For this review, take the finished solid that the model builds, in its own axes (mm). A direction names the side the tool comes from. Give positions to 0.01 mm unless a question says otherwise; leave off trailing zeros. Write each loop counter-clockwise with the first axis right and the second up, starting at its lowest first coordinate (ties: lowest second). Pieces come first, ordered by that corner, then holes. Notation, with made-up numbers: (87, 16.5) -> (111, 16.5) arc R21 ccw to (111, 21.5) -> close; hole circle Ø11 at (25.5, 22). An arc over 180 degrees is marked (long way). Return JSON: item names as keys, results as strings.
from build123d import *

# Parameters (mm, degrees)
SKETCH1_R           = 2.5
BOSS_EXTRUDE1_DEPTH = 283


with BuildPart() as part:
    # Sketch1 → Boss-Extrude1 (new body)
    with BuildSketch(Plane.XY):
        with BuildLine():
            Line((14.316619525, 10.387216168), (13.029112559, 10.387216168))
            Line((13.029112559, 10.387216168), (13.029112559, 12.855371932))
            Line((13.029112559, 12.855371932), (11.656738465, 12.855371932))
            Line((11.656738465, 12.855371932), (11.656738465, 12.336659272))
            Line((11.656738465, 12.336659272), (11.229112559, 12.336659272))
            Line((11.229112559, 12.336659272), (11.229112559, 7.521203168))
            ThreePointArc((11.229112559, 7.521203168), (11.668452387, 6.460542996), (12.729112559, 6.021203168))
            Line((12.729112559, 6.021203168), (17.624436699, 6.021203168))
            Line((17.624436699, 6.021203168), (17.624436699, 6.382997838))
            Line((17.624436699, 6.382997838), (18.129112559, 6.382997838))
            Line((18.129112559, 6.382997838), (18.129112559, 7.755371932))
            Line((18.129112559, 7.755371932), (15.794230869, 7.755371932))
            Line((15.794230869, 7.755371932), (15.794230869, 9.042878898))
            Line((15.794230869, 9.042878898), (18.806723903, 12.055371932))
            Line((18.806723903, 12.055371932), (23.784775289, 12.055371932))
            Line((23.784775289, 12.055371932), (26.797268323, 9.042878898))
            Line((26.797268323, 9.042878898), (26.797268323, 7.755371932))
            Line((26.797268323, 7.755371932), (24.329112559, 7.755371932))
            Line((24.329112559, 7.755371932), (24.329112559, 6.382997838))
            Line((24.329112559, 6.382997838), (24.847825219, 6.382997838))
            Line((24.847825219, 6.382997838), (24.847825219, 6.021203168))
            Line((24.847825219, 6.021203168), (29.729112559, 6.021203168))
            ThreePointArc((29.729112559, 6.021203168), (30.789772731, 6.460542996), (31.229112559, 7.521203168))
            Line((31.229112559, 7.521203168), (31.229112559, 12.350696072))
            Line((31.229112559, 12.350696072), (30.801486653, 12.350696072))
            Line((30.801486653, 12.350696072), (30.801486653, 12.855371932))
            Line((30.801486653, 12.855371932), (29.429112559, 12.855371932))
            Line((29.429112559, 12.855371932), (29.429112559, 10.520490242))
            Line((29.429112559, 10.520490242), (28.141605593, 10.520490242))
            Line((28.141605593, 10.520490242), (25.129112559, 13.532983276))
            Line((25.129112559, 13.532983276), (25.129112559, 18.511034662))
            Line((25.129112559, 18.511034662), (28.141605593, 21.523527696))
            Line((28.141605593, 21.523527696), (29.429112559, 21.523527696))
            Line((29.429112559, 21.523527696), (29.429112559, 19.055371932))
            Line((29.429112559, 19.055371932), (30.801486653, 19.055371932))
            Line((30.801486653, 19.055371932), (30.801486653, 19.574084592))
            Line((30.801486653, 19.574084592), (31.229112559, 19.574084592))
            Line((31.229112559, 19.574084592), (31.229112559, 24.389540696))
            ThreePointArc((31.229112559, 24.389540696), (30.789772731, 25.450200868), (29.729112559, 25.889540696))
            Line((29.729112559, 25.889540696), (24.833788419, 25.889540696))
            Line((24.833788419, 25.889540696), (24.833788419, 25.527746026))
            Line((24.833788419, 25.527746026), (24.329112559, 25.527746026))
            Line((24.329112559, 25.527746026), (24.329112559, 24.155371932))
            Line((24.329112559, 24.155371932), (26.663994249, 24.155371932))
            Line((26.663994249, 24.155371932), (26.663994249, 22.867864966))
            Line((26.663994249, 22.867864966), (23.651501215, 19.855371932))
            Line((23.651501215, 19.855371932), (18.673449829, 19.855371932))
            Line((18.673449829, 19.855371932), (15.660956795, 22.867864966))
            Line((15.660956795, 22.867864966), (15.660956795, 24.155371932))
            Line((15.660956795, 24.155371932), (18.129112559, 24.155371932))
            Line((18.129112559, 24.155371932), (18.129112559, 25.527746026))
            Line((18.129112559, 25.527746026), (17.610399899, 25.527746026))
            Line((17.610399899, 25.527746026), (17.610399899, 25.889540696))
            Line((17.610399899, 25.889540696), (12.729112559, 25.889540696))
            ThreePointArc((12.729112559, 25.889540696), (11.668452387, 25.450200868), (11.229112559, 24.389540696))
            Line((11.229112559, 24.389540696), (11.229112559, 19.560047792))
            Line((11.229112559, 19.560047792), (11.656738465, 19.560047792))
            Line((11.656738465, 19.560047792), (11.656738465, 19.055371932))
            Line((11.656738465, 19.055371932), (13.029112559, 19.055371932))
            Line((13.029112559, 19.055371932), (13.029112559, 21.390253622))
            Line((13.029112559, 21.390253622), (14.316619525, 21.390253622))
            Line((14.316619525, 21.390253622), (17.329112559, 18.377760588))
            Line((17.329112559, 18.377760588), (17.329112559, 13.399709202))
            Line((17.329112559, 13.399709202), (14.316619525, 10.387216168))
        make_face()
        with Locations((21.229112559, 15.955371932)):
            Circle(SKETCH1_R, mode=Mode.SUBTRACT)
    extrude(amount=BOSS_EXTRUDE1_DEPTH)


solid = part.part
1. Add section A-A, the plane x = 21.25. State the section outline as (y, z) points, plus the area to 3 significant figures.
Results found:
{"outline": "(12.06, 0) -> (13.46, 0) -> (13.46, 283) -> (12.06, 283) -> close; (18.46, 0) -> (19.86, 0) -> (19.86, 283) -> (18.46, 283) -> close", "area": "792 mm²"}
2. To check wall thickness, follow probe 1 along X at (y, z) = (20, 163); probe 2 along Y at (x, z) = (21.75, 103); probe 3 along X at (y, z) = (11.5, 155). State the ranges of each line that lie inside material, in increasing order.
Results found:
{"probe 1": "x = 11.23 to 13.03, 15.71 to 18.53, 23.8 to 26.62, 29.43 to 31.23", "probe 2": "y = 12.06 to 13.51, 18.4 to 19.86", "probe 3": "x = 11.23 to 13.03, 15.43 to 18.25, 24.34 to 27.16, 29.43 to 31.23"}
3. For pin 1 (0.7 mm diameter, centred on y = 7, z = 97, fed in from +X); pin 2 (1.5 mm diameter, centred on x = 21.5, z = 148.5, fed in from -Y); pin 3 (0.5 mm diameter, centred on x = 11.5, z = 195, fed in from -Y), all flat-tipped, find the tip position at first contact; note any pin that passes through.
Results found:
{"pin 1": "stops at x = 31.22", "pin 2": "stops at y = 12.06", "pin 3": "stops at y = 6.38"}
4. The part is to be moulded in two halves that separate along X. For faces 6 (the flat face through (31.229, 10, 140)), 7 (the flat face through (21, 19.855, 140)), 8 (the flat face through (23.3, 13.9, 0)), 9 (the flat face through (11.229, 10, 140)), say which applies: +X half, -X half, draft (parallel to the pull), parting line (faces both ways), or undercut.
Results found:
{"face 6": "+X half", "face 7": "undercut", "face 8": "draft", "face 9": "-X half"}
5. For faces 1 (the flat face through (21, 12.055, 140)), 2 (the flat face through (17.329, 16, 140)), 3 (the flat face through (25.129, 16, 140)), 4 (the flat face through (23.3, 13.9, 283)), 5 (the flat face through (31.229, 22, 140)), list the 3-axis set-ups (+Z, -Z, +X, -X, +Y, -Y) from which the entire face can be reached by the end or side of a thin tool; tool diameter is ignored.
Results found:
{"face 1": "+Z, -Z, -Y", "face 2": "+Z, -Z, -X", "face 3": "+Z, -Z, +X", "face 4": "+Z, +X, -X, +Y, -Y", "face 5": "+Z, -Z, +X, +Y, -Y"}
